```python
from build123d import *

# Parameters (mm, degrees)
SKETCH1_W           = 24
SKETCH1_H           = 44
SKETCH1_W_2         = 20.4
SKETCH1_H_2         = 40.4
EXTRUDE_THIN1_DEPTH = 28.4
SKETCH1_2_W         = 20.4
SKETCH1_2_H         = 40.4
BOSS_EXTRUDE1_DEPTH = 2
SKETCH3_W           = 11.27257677
SKETCH3_H           = 19.344298407
CUT_EXTRUDE1_DEPTH  = 25.2


with BuildPart() as part:
    # Sketch1 → Extrude-Thin1 (new body)
    with BuildSketch(Plane(origin=(0, 0, 0), x_dir=(1, 0, 0), z_dir=(0, 1, 0))):
        Rectangle(SKETCH1_W, SKETCH1_H)
        Rectangle(SKETCH1_W_2, SKETCH1_H_2, mode=Mode.SUBTRACT)
    extrude(amount=EXTRUDE_THIN1_DEPTH)

    # Sketch1<2> → Boss-Extrude1 (add)
    with BuildSketch(Plane(origin=(0, 0, 0), x_dir=(1, 0, 0), z_dir=(0, 1, 0))):
        Rectangle(SKETCH1_2_W, SKETCH1_2_H)
    extrude(amount=BOSS_EXTRUDE1_DEPTH)

    # Sketch3 → Cut-Extrude1 (cut)
    with BuildSketch(Plane(origin=(0, 28.4, 0), x_dir=(1, 0, 0), z_dir=(0, 1, 0))):
        with Locations((0, -24.608973671)):
            Rectangle(SKETCH3_W, SKETCH3_H)
    extrude(amount=-CUT_EXTRUDE1_DEPTH, mode=Mode.SUBTRACT)


solid = part.part
```
Part model, mm, in its own coordinate system. A direction names the side the tool comes from. Round coordinates to 2 decimals unless told otherwise and drop trailing zeros. Write each loop counter-clockwise with the first axis right and the second up, starting at its lowest first coordinate (ties: lowest second). Pieces come first, ordered by that corner, then holes. Notation, with made-up numbers: M 44.5,-21 L 102.5,-21 A21 cw 102.5,6 Z; hole C 79,36.5 d8. An arc over 180 degrees is marked long. Answer as CSV lines item,"result". Start each with the question number.
1) Mould opens along Z. For faces 4 (the face through (-10.2, 15, 0)), 5 (the face through (0, 14, -22)), 6 (the face through (0, 3.2, 21)), 7 (the face through (0, 15, -20.2)) say: +Z half, -Z half, draft (parallel to the pull), parting line (faces both ways), or undercut.
2) Band-saw the part on A-A (y = 4.25). List the corners of the cut face in (x, z).
3) Drill centre lines: L1, parallel to X at y = 7, z = 17; L2, parallel to Z at x = -8.25, y = 10; L3, parallel to Z at x = 5.5, y = 7.75. Where is each one in solid material? Low to high.
4) Band-saw the part on C-C (x = 6.75). List the corners of the cut face in (y, z), then the cut area to 3 significant figures.
5) Which spindle directions (+Z, -Z, +X, -X, +Y, -Y) get a long thin tool onto all of the face, cutting with end or side? Do faces 1 (the face through (12, 14, 0)), 2 (the face through (-5.636, 16, 21)), 3 (the face through (10.2, 15, 0)). Say none if no direction does.
6) Drop flat-ended pins along their axis: pin 1 (2 mm diameter, centred on x = 6.5, z = 7.5, fed in from -Y); pin 2 (3 mm diameter, centred on x = 0.5, y = 20, fed in from +Z); pin 3 (8 mm diameter, centred on x = -6, z = 5.5, fed in from +Y); pin 4 (0.9 mm diameter, centred on x = 2, z = 21, fed in from +Y). Give the stop position or say it passes through.
7) Band-saw the part on B-B (z = 0). List the corners of the cut face in (x, y), then the cut area to 3 significant figures.
Worked out:
1,face 4,"undercut"
1,face 5,"-Z half"
1,face 6,"draft"
1,face 7,"undercut"
2,outline,"M -12,-22 L 12,-22 L 12,22 L 5.64,22 L 5.64,20.2 L 10.2,20.2 L 10.2,-20.2 L -10.2,-20.2 L -10.2,20.2 L -5.64,20.2 L -5.64,22 L -12,22 Z"
3,L1,"-12 to -10.2, 10.2 to 12"
3,L2,"-22 to -20.2, 20.2 to 22"
3,L3,"-22 to -20.2"
4,outline,"M 0,-22 L 28.4,-22 L 28.4,-20.2 L 2,-20.2 L 2,20.2 L 28.4,20.2 L 28.4,22 L 0,22 Z"
4,area,"183 mm²"
5,face 1,"+Z, -Z, +X, +Y, -Y"
5,face 2,"+Z, +Y"
5,face 3,"+Y"
6,pin 1,"y = 0"
6,pin 2,"z = -20.2"
6,pin 3,"y = 2"
6,pin 4,"y = 3.2"
7,outline,"M -12,0 L 12,0 L 12,28.4 L 10.2,28.4 L 10.2,2 L -10.2,2 L -10.2,28.4 L -12,28.4 Z"
7,area,"143 mm²"
